```python
from build123d import *

# Parameters (mm, degrees)
F0_W     = 81.28
F0_H     = 81.28
F1_DEPTH = 35.306
F2_R     = 16.432892
F3_DEPTH = 52.324
F2_R_2   = 21.403736
F4_DEPTH = 55.88


with BuildPart() as f1:
    # F0 (on Front) → F1 (new body)
    with BuildSketch(Plane.XZ):
        Rectangle(F0_W, F0_H)
    extrude(amount=F1_DEPTH)

    # F2 (on Front) → F3 (cut)
    with BuildSketch(Plane.XZ):
        Circle(F2_R)
    extrude(amount=F3_DEPTH, mode=Mode.SUBTRACT)

    # F2 (on Front) → F4 (join)
    with BuildSketch(Plane.XZ):
        Circle(F2_R_2)
        Circle(F2_R, mode=Mode.SUBTRACT)
    extrude(amount=F4_DEPTH)


solid = f1.part
```
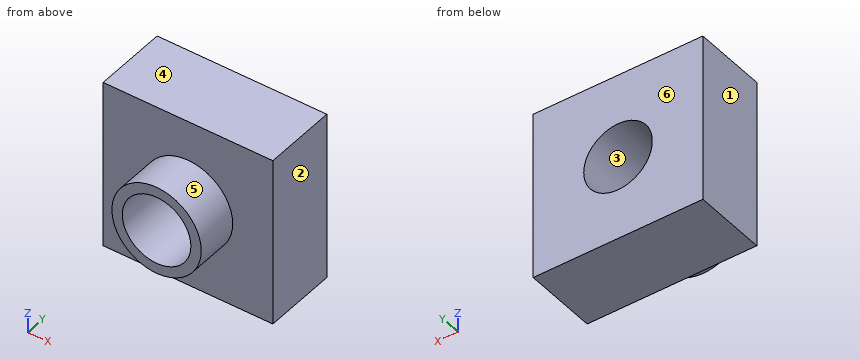
Verification items for the finished model (mm, model axes). Face numbers are marked on the shaded views. A direction names the side the tool comes from. Coordinates: 2 decimals unless noted, no trailing zeros. Loops run counter-clockwise (first coordinate to the right, second up) from the corner with the lowest first, then second, coordinate; pieces in that order, holes last. Notation, with made-up numbers: (-13.5, -3) - (8.5, -3) arc R11 ccw to (8.5, 12) - close; hole circle Ø2 at (-2.75, 81.5). An arc over 180 degrees is marked (long way). Return JSON: item names as keys, results as strings.
1. Section check A-A, the plane x = 0. Record the boundary of the cut face in (y, z).
Established:
{"outline": "(-55.88, -21.4) - (-35.31, -21.4) - (-35.31, -40.64) - (0, -40.64) - (0, -16.43) - (-55.88, -16.43) - close; (-55.88, 16.43) - (0, 16.43) - (0, 40.64) - (-35.31, 40.64) - (-35.31, 21.4) - (-55.88, 21.4) - close"}
2. Mould release check, pull along X, two halves, no side actions. Record for the marked faces 1, 2, 3 and 4: +X half, -X half, draft (parallel to the pull), parting line (faces both ways), or undercut.
Established:
{"face 1": "-X half", "face 2": "+X half", "face 3": "undercut", "face 4": "draft"}
3. Section check B-B, the plane z = 0. Record the boundary of the cut face in (x, y), then the cut area to 3 significant figures.
Established:
{"outline": "(-40.64, -35.31) - (-21.4, -35.31) - (-21.4, -55.88) - (-16.43, -55.88) - (-16.43, 0) - (-40.64, 0) - close; (16.43, -55.88) - (21.4, -55.88) - (21.4, -35.31) - (40.64, -35.31) - (40.64, 0) - (16.43, 0) - close", "area": "1,910 mm2"}
4. Section check D-D, the plane z = 18. Record the boundary of the cut face in (x, y), then the cut area to 3 significant figures.
Established:
{"outline": "(-40.64, -35.31) - (-11.58, -35.31) - (-11.58, -55.88) - (11.58, -55.88) - (11.58, -35.31) - (40.64, -35.31) - (40.64, 0) - (-40.64, 0) - close", "area": "3,350 mm2"}
5. Go/stop test with a flat-tipped pin: pin 1 (2 mm diameter, centred on x = 15, z = 5, fed in from -Y). Record where the tip stops, or that it passes through.
Established:
{"pin 1": "stops at y = -55.88"}
6. Thickness scan on L1, parallel to Z at x = 0, y = -42; L2, parallel to Z at x = 0, y = -23; L3, parallel to Y at x = -28.5, z = 37. Record the ranges inside material, lowest first.
Established:
{"L1": "z = -21.4 to -16.43, 16.43 to 21.4", "L2": "z = -40.64 to -16.43, 16.43 to 40.64", "L3": "y = -35.31 to 0"}
7. Tool access check on the marked faces 5 and 6. Record the directions out of +Z, -Z, +X, -X, +Y, -Y that give a thin tool (end or side, any length) a straight path to the whole face; none if there is none.
Established:
{"face 5": "-Y", "face 6": "+Z, -Z, +X, -X, +Y"}
8. Section check C-C, the plane y = -16. Record the boundary of the cut face in (x, z), then the cut area to 3 significant figures.
Established:
{"outline": "(-40.64, -40.64) - (40.64, -40.64) - (40.64, 40.64) - (-40.64, 40.64) - close; hole circle Ø32.87 at (0, 0)", "area": "5,760 mm2"}
